Here's the drawing with two shaded views (mm, measured from the low corner). I have some questions. Coordinates: 2 decimals unless noted, no trailing zeros. Loops run counter-clockwise (first coordinate to the right, second up) from the corner with the lowest first, then second, coordinate; pieces in that order, holes last. Notation, with made-up numbers: M 28.5,2 L 69.5,2 A4 cw 69.5,9 Z; hole C -20,-3.75 d9. An arc over 180 degrees is marked long. Return JSON: item names as keys, results as strings. Group by question number.
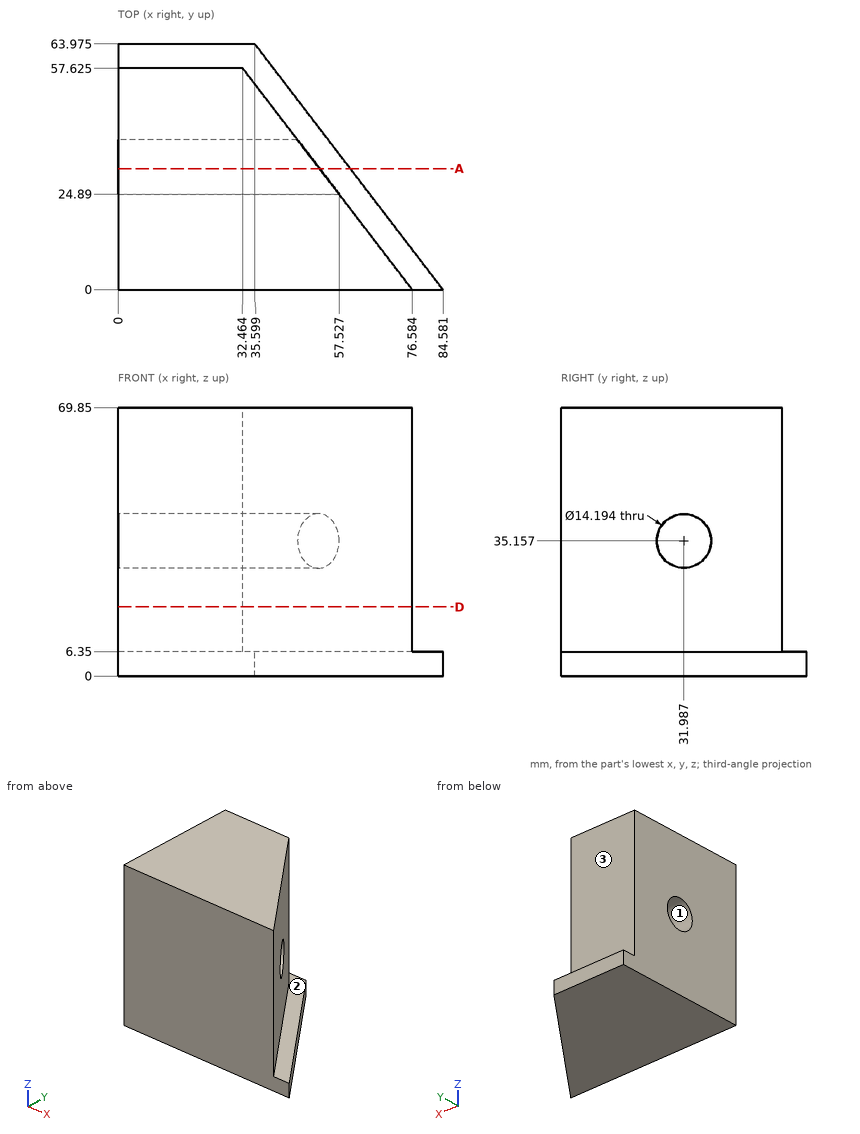
(1) If I drill on L1, parallel to Y at x = 15, z = 25.5 (1 decimal); L2, parallel to Z at x = 54, y = 34.5; L3, parallel to X at y = 40, z = 51, over which ranges is the centre line in solid material (lowest first)? Write a range as [from, to].
(2) Imagine slicing it at A-A, the plane y = 31.5. Write out the boundary of the cut face in (x, z).
(3) Imagine slicing it at D-D, the plane z = 18. Write out the boundary of the cut face in (x, y) (1 decimal), then the cut area to 3 significant figures.
(4) Will these pins go through, and if not, where does the flat tip stop? P1, Ø10, axis at y = 41, z = 35, coming from the +X side; P2, Ø2, axis at y = 17.5, z = 62.5, coming from the -X side; P3, Ø2, axis at y = 12.5, z = 31.5, coming from the +X side; P4, Ø10, axis at x = 9, z = 25, coming from the +Y side (1 decimal).
(5) We'd pull the mould along Y, two halves only. Please class the marked faces 1, 2 and 3: +Y half, -Y half, draft (parallel to the pull), parting line (faces both ways), or undercut.
Checks:
{
 "1": {"L1": "[0, 57.6]", "L2": "[0, 6.35]", "L3": "[0, 45.96]"},
 "2": {"outline": "M 0,0 L 60.46,0 L 60.46,6.35 L 52.47,6.35 L 52.47,28.08 L 0,28.08 Z; M 0,42.24 L 52.47,42.24 L 52.47,69.85 L 0,69.85 Z"},
 "3": {"outline": "M 0,0 L 76.6,0 L 32.5,57.6 L 0,57.6 Z", "area": "3,140 mm²"},
 "4": {"P1": "x = 47.62", "P2": "x = 0", "P3": "x = 67.78", "P4": "y = 57.6"},
 "5": {"face 1": "undercut", "face 2": "draft", "face 3": "+Y half"}
}
